from build123d import *

# Parameters (mm, degrees)
SKETCH1_R           = 2.1
BOSS_EXTRUDE1_DEPTH = 10
SKETCH6_W           = 30
SKETCH6_H           = 30
SKETCH6_W_2         = 20
SKETCH6_H_2         = 20
BOSS_EXTRUDE5_DEPTH = 40
SKETCH7_R           = 4.35
CUT_EXTRUDE1_DEPTH  = 53.92447449
CUT_EXTRUDE2_REACH  = 70.381
SKETCH8_R           = 2.15
FILLET2_R           = 10


# Read off the part's stored shape, not the designer's step: moBlkMgr[demtay]
with BuildPart() as part:
    # Sketch1 → Boss-Extrude1 (new body)
    with BuildSketch(Plane(origin=(0, 0, 0), x_dir=(1, 0, 0), z_dir=(0, 1, 0))):
        with BuildLine():
            Line((-14, 25), (14, 25))
            ThreePointArc((14, 25), (21.071067812, 22.071067812), (24, 15))
            Line((24, 15), (24, -15))
            ThreePointArc((24, -15), (21.071067812, -22.071067812), (14, -25))
            Line((14, -25), (-14, -25))
            ThreePointArc((-14, -25), (-21.071067812, -22.071067812), (-24, -15))
            Line((-24, -15), (-24, 15))
            ThreePointArc((-24, 15), (-21.071067812, 22.071067812), (-14, 25))
        make_face()
        with Locations(Location((-18, 18.75, 0), (0, 0, 270))):
            Circle(SKETCH1_R, mode=Mode.SUBTRACT)
        with Locations(Location((18, 18.75, 0), (0, 0, 270))):
            Circle(SKETCH1_R, mode=Mode.SUBTRACT)
        with Locations(Location((18, -18.75, 0), (0, 0, 270))):
            Circle(SKETCH1_R, mode=Mode.SUBTRACT)
        with Locations(Location((-18, -18.75, 0), (0, 0, 270))):
            Circle(SKETCH1_R, mode=Mode.SUBTRACT)
    extrude(amount=BOSS_EXTRUDE1_DEPTH)

    # Sketch6 → Boss-Extrude5 (add)
    with BuildSketch(Plane(origin=(0, 0, 0), x_dir=(-1, 0, 0), z_dir=(0, -1, 0))):
        with Locations((0, -10)):
            Rectangle(SKETCH6_W, SKETCH6_H)
        with Locations((0, -10)):
            Rectangle(SKETCH6_W_2, SKETCH6_H_2, mode=Mode.SUBTRACT)
    extrude(amount=BOSS_EXTRUDE5_DEPTH)

    # Sketch7 → Cut-Extrude1 (cut, through all)
    with BuildSketch(Plane(origin=(0, 0, 0), x_dir=(-1, 0, 0), z_dir=(0, -1, 0))):
        with Locations((-18, -18.75)):
            Circle(SKETCH7_R)
        with Locations((18, -18.75)):
            Circle(SKETCH7_R)
    extrude(amount=CUT_EXTRUDE1_DEPTH, mode=Mode.SUBTRACT)

    # Sketch8 → Cut-Extrude2 (cut, up to next)
    with BuildSketch(Plane.XY.offset(25), mode=Mode.PRIVATE) as cut_extrude2_sk1:
        with Locations((0, -8)):
            Circle(SKETCH8_R)
    cut_extrude2_tool1 = extrude(cut_extrude2_sk1.sketch, amount=-CUT_EXTRUDE2_REACH, mode=Mode.PRIVATE) & part.part
    # Sketch8 → Cut-Extrude2 (cut, up to next)
    with BuildSketch(Plane.XY.offset(25), mode=Mode.PRIVATE) as cut_extrude2_sk2:
        with Locations((0, -28)):
            Circle(SKETCH8_R)
    cut_extrude2_tool2 = extrude(cut_extrude2_sk2.sketch, amount=-CUT_EXTRUDE2_REACH, mode=Mode.PRIVATE) & part.part
    add(cut_extrude2_tool1.solids().sort_by_distance((0, -8, 25))[0], mode=Mode.SUBTRACT)
    add(cut_extrude2_tool2.solids().sort_by_distance((0, -28, 25))[0], mode=Mode.SUBTRACT)

    # Fillet2
    fillet2_edges = [part.edges().sort_by_distance(p)[0] for p in [
        (0, 0, -5),
    ]]
    fillet(fillet2_edges, radius=FILLET2_R)


solid = part.part
Could you check a few things on this model? Use its own coordinates, in mm. A direction names the side the tool comes from. Coordinates: 2 decimals unless noted, no trailing zeros. Write each loop counter-clockwise with the first axis right and the second up, starting at its lowest first coordinate (ties: lowest second). Pieces come first, ordered by that corner, then holes. Notation, with made-up numbers: M 6,36 L 51,36 A16 ccw 51,54 Z; hole C 55.25,15 d9. An arc over 180 degrees is marked long. One line per question, with ' | ' between items.
1) Imagine slicing it at B-B, the plane x = 0. Write out the boundary of the cut face in (y, z).
Checks:
outline: M -40,-5 L -10,-5 A10 cw 0,-15 L 0,-25 L 10,-25 L 10,25 L -5.85,25 L -5.85,20 L 0,20 L 0,0 L -40,0 Z; M -40,20 L -30.15,20 L -30.15,25 L -40,25 Z; M -25.85,20 L -10.15,20 L -10.15,25 L -25.85,25 Z
2) If we mould it in two halves opening along X, with no side actions, what happens to faces 6 (the face through (13.65, -19.72, 18.8)), 7 (the face through (-0.28, -5.87, 22.54)), 8 (the face through (10.2, -40, 9.8))? For each: released by +X, released by -X, zero draft, split by the parting line, or undercut.
Checks:
face 6: released by +X | face 7: undercut | face 8: zero draft
3) For pin 1 Ø10 at (x, z) = (3.5, 10.5) entering from -Y; pin 2 Ø3.5 at (x, y) = (0, -28) entering from -Z; pin 3 Ø24.5 at (y, z) = (-23.5, -1.5) entering from +X, each with a flat end and sliding along its axis, tell me the tip position at first contact or that it passes through.
Checks:
pin 1: y = 0 | pin 2: z = -5 | pin 3: x = 15
4) Imagine slicing it at A-A, the plane y = -32.5. Write out the boundary of the cut face in (x, z), and give its area (3 significant figures).
Checks:
outline: M -15,-5 L 15,-5 L 15,15.6 A4.35 cw 15,21.9 L 15,25 L -15,25 L -15,21.9 A4.35 cw -15,15.6 Z; hole M -10,0 L 10,0 L 10,20 L -10,20 Z | area: 488 mm²
5) Imagine slicing it at D-D, the plane x = -9. Write out the boundary of the cut face in (y, z), and give its area (3 significant figures).
Checks:
outline: M -40,-5 L -10,-5 A10 cw 0,-15 L 0,-25 L 10,-25 L 10,25 L -40,25 L -40,20 L 0,20 L 0,0 L -40,0 Z | area: 921 mm²
6) I need wall thicknesses on probe 1 along Y at (x, z) = (0, 21); probe 2 along Z at (x, y) = (8, -32.5); probe 3 along X at (y, z) = (5, 18.75). Which ranges of each line are inside material? Lowest first, please. Write a range as [from, to].
Checks:
probe 1: [-40, -30.15], [-25.85, -10.15], [-5.85, 10] | probe 2: [-5, 0], [20, 25] | probe 3: [-23.27, -20.1], [-15.9, 15.9], [20.1, 23.27]
7) Imagine slicing it at C-C, the plane z = -18.75. Write out the boundary of the cut face in (x, y).
Checks:
outline: M -23.27,0 L -20.1,0 L -20.1,10 L -23.27,10 Z; M -15.9,0 L 15.9,0 L 15.9,10 L -15.9,10 Z; M 20.1,0 L 23.27,0 L 23.27,10 L 20.1,10 Z
8) For faces 1 (the face through (0, -20, 0)), 2 (the face through (15, -20, 23)), 3 (the face through (-0.47, -30.1, 22.54)), 4 (the face through (0, 5, -25)), 5 (the face through (-15, -20, 4)), which set-ups out of +Z, -Z, +X, -X, +Y, -Y let a thin tool reach every point of the face, with its end or its side?
Checks:
face 1: -Y | face 2: +Z, -Z, +X, -Y | face 3: +Z | face 4: -Z, +X, -X, +Y, -Y | face 5: +Z, -Z, -X, -Y
